Verification items for this drawing (mm, ordinates from the low corner). A direction names the side the tool comes from. Round coordinates to 2 decimals unless told otherwise and drop trailing zeros. Order: outer loops, then holes, each group sorted by start corner. A loop starts at its lowest first (then second) coordinate and runs counter-clockwise, first axis right, second up. Notation, with made-up numbers: (18.25, 76.25) -> (68.25, 76.25) arc R19 cw to (68.25, 104.25) -> close; hole circle Ø4 at (-11, 50.25). An arc over 180 degrees is marked (long way). Return JSON: item names as keys, results as strings. Group by question number.
Item 1: Sectioned sample at A-A on x = 4. Record the cut outline in (y, z), plus the area to 3 significant figures.
Item 2: Sectioned sample at B-B on z = 4. Record the cut outline in (x, y).
Item 3: Access from +Z, -Z, +X, -X, +Y, -Y to the whole of each face (thin tool, end or side, straight path). Record for the marked faces 1, 2 and 3.
Item 4: Draft check along Z on the marked faces 4, 5, 6 and 7. Enter one of: pulls with the +Z half, pulls with the -Z half, needs draft (parallel to the pull), parting line crosses it, or undercut.
Item 5: Scan lines: probe 1 along X at (y, z) = (0.35, 2); probe 2 along Y at (x, z) = (0.75, 1.75); probe 3 along Y at (x, z) = (2, 2). Record each from-to range of solid material in increasing order. Write a range as from..to.
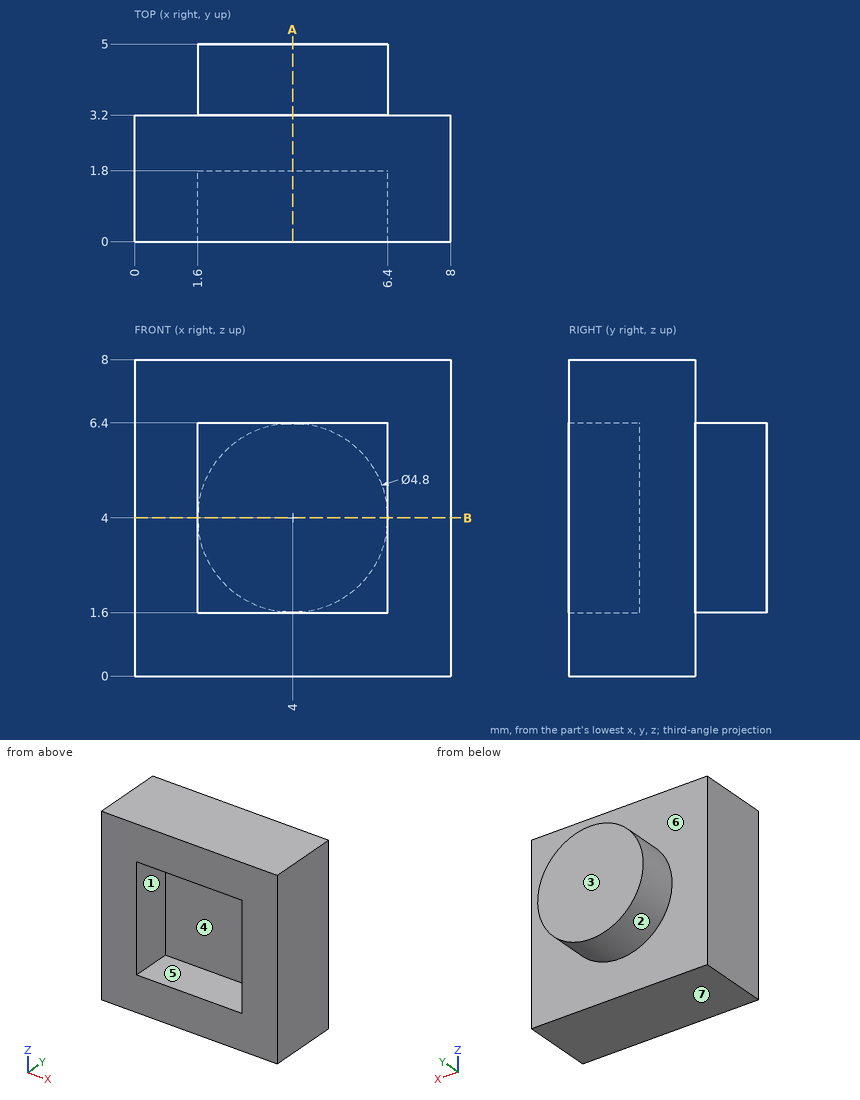
Recorded:
{
 "1": {"outline": "(0, 0) -> (3.2, 0) -> (3.2, 1.6) -> (5, 1.6) -> (5, 6.4) -> (3.2, 6.4) -> (3.2, 8) -> (0, 8) -> (0, 6.4) -> (1.8, 6.4) -> (1.8, 1.6) -> (0, 1.6) -> close", "area": "25.6 mm²"},
 "2": {"outline": "(0, 0) -> (1.6, 0) -> (1.6, 1.8) -> (6.4, 1.8) -> (6.4, 0) -> (8, 0) -> (8, 3.2) -> (6.4, 3.2) -> (6.4, 5) -> (1.6, 5) -> (1.6, 3.2) -> (0, 3.2) -> close"},
 "3": {"face 1": "-Y", "face 2": "+Y", "face 3": "+Z, -Z, +X, -X, +Y"},
 "4": {"face 4": "undercut", "face 5": "undercut", "face 6": "needs draft", "face 7": "pulls with the -Z half"},
 "5": {"probe 1": "0..1.6, 6.4..8", "probe 2": "0..3.2", "probe 3": "1.8..3.2"}
}
